Design review of the part built by this model. Coordinates are the model's own, in mm. Coordinates: 2 decimals unless noted, no trailing zeros. Write each loop counter-clockwise with the first axis right and the second up, starting at its lowest first coordinate (ties: lowest second). Pieces come first, ordered by that corner, then holes. Notation, with made-up numbers: M 71,-37 L 128,-37 A22 cw 128,-4 Z; hole C 35,31 d6. An arc over 180 degrees is marked long. One line per question, with ' | ' between items.
from build123d import *

# Parameters (mm, degrees)
CORTAR_EXTRUIR1_DEPTH = 51


with BuildPart() as part:
    # Croquis1 → Revolución1 (revolve)
    with BuildSketch(Plane.XY):
        Polygon((0, 0), (-48.25, 0), (-48.25, 13.3), (-8.5, 48), (0, 50), align=None)
    revolve(axis=Axis((0, 53.503350084, 0), (0, -1, 0)))

    # Croquis2 → Cortar-Extruir1 (cut, through all)
    with BuildSketch(Plane.XZ):
        with BuildLine():
            ThreePointArc((41.268177813, 25), (0, 48.25), (-41.268177813, 25))
            Line((-41.268177813, 25), (41.268177813, 25))
        make_face()
        with BuildLine():
            Line((41.268177813, -25), (-41.268177813, -25))
            ThreePointArc((-41.268177813, -25), (0, -48.25), (41.268177813, -25))
        make_face()
    extrude(amount=-CORTAR_EXTRUIR1_DEPTH, mode=Mode.SUBTRACT)


solid = part.part
1. To check wall thickness, follow line 1 along X through (y, z) = (8, 0.5); line 2 along Y through (x, z) = (10.5, 17.5); line 3 along Y through (x, z) = (13, -14.5). State the ranges of each line that lie inside material, in increasing order. Write a range as [from, to].
Answer sheet:
line 1: [-48.25, 48.25] | line 2: [0, 37.6] | line 3: [0, 38.42]
2. Take a section at B-B (y = 35.5). Write out the cut boundary in (x, z), then the cut area to 3 significant figures.
Answer sheet:
outline: C 0,0 d45.64 | area: 1,640 mm^2
3. Take a section at A-A (y = 7.5). Write out the cut boundary in (x, z), then the cut area to 3 significant figures.
Answer sheet:
outline: M -41.27,-25 L 41.27,-25 A48.25 ccw 41.27,25 L -41.27,25 A48.25 ccw Z | area: 4,600 mm^2
4. Insertion check: pin 1 Ø3 at (y, z) = (32, 19.5) entering from -X; pin 2 Ø5 at (x, y) = (-36.5, 29.5) entering from +Z. Each pin has a flat end and moves straight along its axis. Give the tip position at first contact, or say it passes through.
Answer sheet:
pin 1: x = -21.22 | pin 2: through
